Could you check a few things on this drawing? It's one solid part, dimensions in mm from its lowest x, y, z. Give positions to 0.01 mm unless a question says otherwise; leave off trailing zeros. Loops run counter-clockwise (first coordinate to the right, second up) from the corner with the lowest first, then second, coordinate; pieces in that order, holes last. Notation, with made-up numbers: M 46,45 L 98,45 A17 cw 98,76 Z; hole C -12.75,11 d10. An arc over 180 degrees is marked long. Return JSON: item names as keys, results as strings. Group by question number.
1. Please list where these lines run through material, in increasing order: line 1 (Z direction, x = 49.5, y = 2.7) (3 decimals); line 2 (X direction, y = 2.55, z = 101) (3 decimals); line 3 (Z direction, x = 47, y = 2.5) (3 decimals).
2. If we section it at B-B (y = 2.35): State how many separate pieces and enclosed holes the cut face has, plus the area to 3 significant figures.
3. If we section it at A-A (x = 50.8): Write out the boundary of the cut face in (y, z) (3 decimals).
4. For pin 1 (1 mm diameter, centred on y = 1.5, z = 105.5, fed in from -X) (3 decimals); pin 2 (1 mm diameter, centred on x = 79, y = 0.5, fed in from -Z); pin 3 (1 mm diameter, centred on x = 14, y = 1, fed in from +Z), each with a flat end and sliding along its axis, tell me the tip position at first contact or that it passes through.
5. If we section it at C-C (x = 70): Write out the boundary of the cut face in (y, z) (3 decimals).
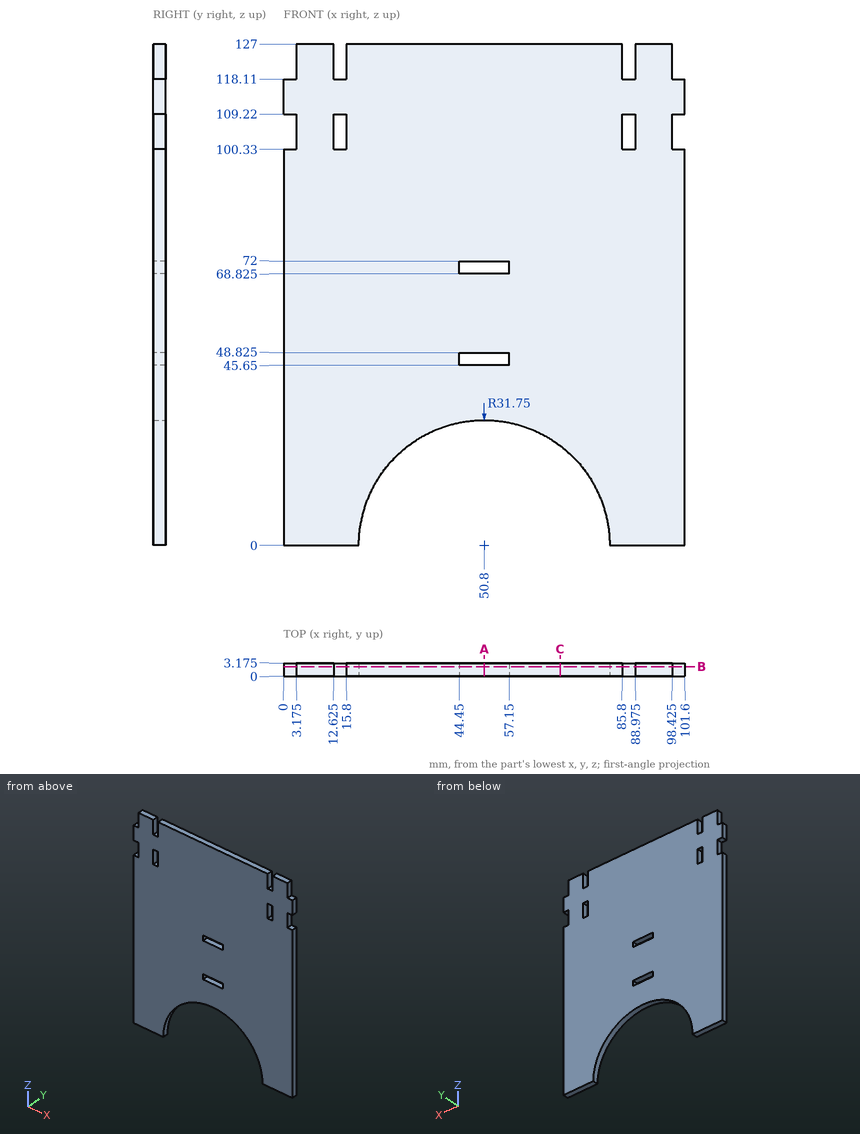
Answer:
{
 "1": {"line 1": "z = 31.723 to 45.65, 48.825 to 68.825, 72 to 127", "line 2": "x = 3.175 to 12.625, 15.8 to 85.8, 88.975 to 98.425", "line 3": "z = 31.522 to 45.65, 48.825 to 68.825, 72 to 127"},
 "2": {"separate pieces": "1", "enclosed holes": "4", "area": "11,000 mm²"},
 "3": {"outline": "M 0,31.75 L 3.175,31.75 L 3.175,45.65 L 0,45.65 Z; M 0,48.825 L 3.175,48.825 L 3.175,68.825 L 0,68.825 Z; M 0,72 L 3.175,72 L 3.175,127 L 0,127 Z"},
 "4": {"pin 1": "stops at x = 3.175", "pin 2": "stops at z = 13.58", "pin 3": "stops at z = 118.11"},
 "5": {"outline": "M 0,25.287 L 3.175,25.287 L 3.175,127 L 0,127 Z"}
}
